```python
from build123d import *

# Parameters (mm, degrees)
F2_SIZE  = 0.5
F3_R     = 23.5
F4_DEPTH = 30
F5_SIZE  = 1


with BuildPart() as f1:
    # F0 (on Right) → F1 (revolve)
    with BuildSketch(Plane.YZ):
        Polygon((-40.5099816322, 9), (3.4900183678, 9), (3.4900183678, 50), (-0.5099816322, 50), (-16.0099816322, 34.5), (-16.0099816322, 32), (-21.0099816322, 32), (-21.0099816322, 34.5), (-36.5099816322, 50), (-40.5099816322, 50), align=None)
    revolve(axis=Axis((0, -20.3511445433, 0), (0, 1, 0)))

    # F2
    f2_edges = [f1.edges().sort_by_distance(p)[0] for p in [
        (0, -40.509982, -9),
        (0, -40.509982, -50),
        (0, 3.490018, -50),
        (0, 3.490018, -9),
    ]]
    chamfer(f2_edges, length=F2_SIZE)

    # F3 (on face) → F4 (cut)
    with BuildSketch(Plane.XZ.offset(40.5099816322)):
        Circle(F3_R)
    extrude(amount=-F4_DEPTH, mode=Mode.SUBTRACT)

    # F5
    f5_edges = [f1.edges().sort_by_distance(p)[0] for p in [
        (-23.5, -40.509982, 0),
        (0, -10.509982, -9),
        (-23.5, -10.509982, 0),
    ]]
    chamfer(f5_edges, length=F5_SIZE)


solid = f1.part
```
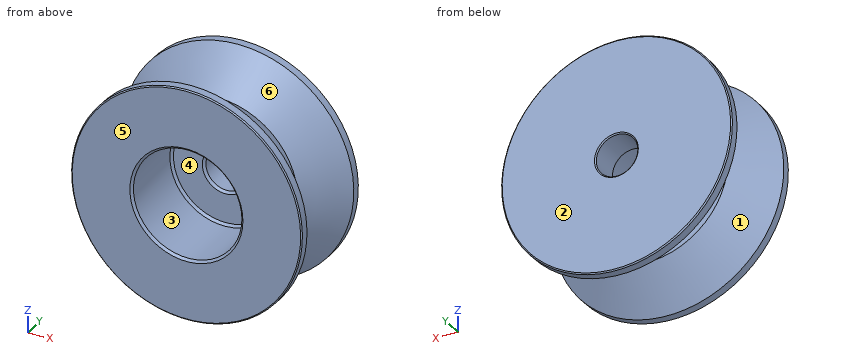
Check sheet for the modelled part. Datum: model origin and axes. Units: mm. Face numbers are marked on the shaded views. A direction names the side the tool comes from. Give positions to 0.01 mm unless a question says otherwise; leave off trailing zeros. Loops run counter-clockwise (first coordinate to the right, second up) from the corner with the lowest first, then second, coordinate; pieces in that order, holes last. Notation, with made-up numbers: M -10.75,76.25 L -4.75,76.25 A23 cw -4.75,106.25 Z; hole C 48.25,17 d3. An arc over 180 degrees is marked long. Answer in a Markdown table with one row per item.
1) Thickness scan on line 1 (X direction, y = 0, z = 0); line 2 (Y direction, x = 15.5, z = 30); line 3 (Z direction, x = 0, y = -24). Record the ranges inside material, lowest first.
Solutions:
| item | result |
|---|---|
| line 1 | x = -50 to -9, 9 to 50 |
| line 2 | y = -40.51 to -21.01, -16.01 to 3.49 |
| line 3 | z = -37.49 to -23.5, 23.5 to 37.49 |
2) Cross-section at A-A (y = -19). Enter the section's corners in (x, z).
Solutions:
| item | result |
|---|---|
| outline | C 0,0 d64; hole C 0,0 d47 |
3) Cross-section at B-B (y = -8). Enter the section's corners in (x, z), plus the area to 3 significant figures.
Solutions:
| item | result |
|---|---|
| outline | C 0,0 d85.02; hole C 0,0 d18 |
| area | 5,420 mm^2 |
4) Tool access check on the marked faces 1, 2 and 3. Record the directions out of +Z, -Z, +X, -X, +Y, -Y that give a thin tool (end or side, any length) a straight path to the whole face; none if there is none.
Solutions:
| item | result |
|---|---|
| face 1 | none |
| face 2 | +Z, -Z, +X, -X, +Y |
| face 3 | -Y |
5) Depth check by flat-ended pin: pin 1 (6 mm diameter, centred on y = -7.5, z = 33, fed in from +X); pin 2 (11 mm diameter, centred on x = 0, z = 0, fed in from +Y); pin 3 (4 mm diameter, centred on x = 9.5, y = -13.5, fed in from +Z); pin 4 (8 mm diameter, centred on y = -14, z = -14, fed in from -X). Enter the tip coordinate at first touch or a pass-through.
Solutions:
| item | result |
|---|---|
| pin 1 | stops at x = 33 |
| pin 2 | passes through |
| pin 3 | stops at z = 37.89 |
| pin 4 | stops at x = -38.24 |
6) Mould release check, pull along X, two halves, no side actions. Record for the marked faces 4, 5 and 6: released by +X, released by -X, zero draft, split by the parting line, or undercut.
Solutions:
| item | result |
|---|---|
| face 4 | undercut |
| face 5 | zero draft |
| face 6 | split by the parting line |
